from build123d import *

# Parameters (mm, degrees)
SKETCH1_R           = 8.5
SKETCH1_R_2         = 1.5
BOSS_EXTRUDE1_DEPTH = 3
FILLET1_R           = 3


with BuildPart() as part:
    # Sketch1 → Boss-Extrude1 (new body)
    with BuildSketch(Plane(origin=(0, 0, 0), x_dir=(1, 0, 0), z_dir=(0, 1, 0))):
        Polygon((-11, 0), (11, 0), (20.489621783, 17.605313925), (20.489621783, 47.605313925), (8, 62), (-8, 62), (-20.509243816, 47.910305032), (-20.509243816, 17.610706132), align=None)
        with Locations((7.519679741, 17.780252273)):
            Circle(SKETCH1_R, mode=Mode.SUBTRACT)
        with Locations((6, 4)):
            Circle(SKETCH1_R_2, mode=Mode.SUBTRACT)
        with Locations((-6, 4)):
            Circle(SKETCH1_R_2, mode=Mode.SUBTRACT)
        with Locations((-5.25, 57.999859765)):
            Circle(SKETCH1_R_2, mode=Mode.SUBTRACT)
        with Locations((5.25, 57.999859765)):
            Circle(SKETCH1_R_2, mode=Mode.SUBTRACT)
        with Locations((-13.5, 37.605313925)):
            Circle(SKETCH1_R_2, mode=Mode.SUBTRACT)
        with Locations((13.5, 37.605313925)):
            Circle(SKETCH1_R_2, mode=Mode.SUBTRACT)
        with BuildLine():
            Line((-8.730303993, 39.105313925), (8.730303993, 39.105313925))
            ThreePointArc((8.730303993, 39.105313925), (10.179901517, 41.34388933), (12.574074074, 42.518832133))
            ThreePointArc((12.574074074, 42.518832133), (0, 51.105313925), (-12.574074074, 42.518832133))
            ThreePointArc((-12.574074074, 42.518832133), (-10.179901517, 41.34388933), (-8.730303993, 39.105313925))
        make_face(mode=Mode.SUBTRACT)
        with BuildLine():
            Line((-8.730303993, 36.105313925), (8.730303993, 36.105313925))
            ThreePointArc((8.730303993, 36.105313925), (9.667400631, 34.394210987), (11.187975781, 33.171969363))
            ThreePointArc((11.187975781, 33.171969363), (11.998189223, 31.105465162), (10.062695821, 30.018841621))
            ThreePointArc((10.062695821, 30.018841621), (-0.366780245, 27.478383479), (-4.980318958, 17.785955551))
            ThreePointArc((-4.980318958, 17.785955551), (-9.241131059, 13.528058523), (-13.5, 17.787899155))
            Line((-13.5, 17.787899155), (-13.5, 32.605313925))
            ThreePointArc((-13.5, 32.605313925), (-10.541960108, 33.574185051), (-8.730303993, 36.105313925))
        make_face(mode=Mode.SUBTRACT)
    extrude(amount=BOSS_EXTRUDE1_DEPTH)

    # Fillet1
    fillet1_edges = [part.edges().sort_by_distance(p)[0] for p in [
        (-20.509243816, 1.5, -17.610706132),
        (-20.509243816, 1.5, -47.910305032),
        (-8, 1.5, -62),
        (8, 1.5, -62),
        (20.489621783, 1.5, -47.605313925),
        (20.489621783, 1.5, -17.605313925),
    ]]
    fillet(fillet1_edges, radius=FILLET1_R)


solid = part.part
The model under review builds one solid part; all positions refer to its coordinate system, in mm. A direction names the side the tool comes from. Round coordinates to 2 decimals unless told otherwise and drop trailing zeros. Order: outer loops, then holes, each group sorted by start corner. A loop starts at its lowest first (then second) coordinate and runs counter-clockwise, first axis right, second up. Notation, with made-up numbers: (-25.75, 43.5) -> (10.25, 43.5) arc R17 cw to (10.25, 62.5) -> close; hole circle Ø11 at (62, 18). An arc over 180 degrees is marked (long way). Write item = value, one per line. Start each with the question number.
Item 1: Consider section D-D on y = 1.3. Count the separate pieces of the cut face and the enclosed holes in it, plus the area to 3 significant figures.
Item 2: For faces 1 (the face through (0, 1, -62)), 2 (the face through (-0.246, 1.479, -27.576)), list the 3-axis set-ups (+Z, -Z, +X, -X, +Y, -Y) from which the entire face can be reached by the end or side of a thin tool; tool diameter is ignored.
Item 3: Consider section A-A on z = -4. Write out the cut boundary in (x, y).
Item 4: Consider section C-C on z = -12.5. Write out the cut boundary in (x, y).
Item 5: For line 1 along Z through (x, y) = (1.5, 0.5); line 2 along Z through (x, y) = (11.5, 0.55); line 3 along X through (y, z) = (1.7, -25), list the stretches that pass through material, from the lowest coordinate up.
Item 6: Consider section B-B on x = -6. Write out the cut boundary in (y, z).
Item 7: Mouldability with a two-part tool opening along X and no side actions: class faces 3 (the face through (0, 3, -38)), 4 (the face through (-10.578, 1.479, -33.548)), 5 (the face through (-20.415, 1.521, -17.624)) as released by +X, released by -X, zero draft, split by the parting line, or undercut.
Conclusion:
q1.separate_pieces = 1
q1.enclosed_holes = 9
q1.area = 1,400 mm2
q2.face_1 = -Z, +X, -X, +Y, -Y
q2.face_2 = +Y, -Y
q3.outline = (-13.16, 0) -> (-7.5, 0) -> (-7.5, 3) -> (-13.16, 3) -> close; (-4.5, 0) -> (4.5, 0) -> (4.5, 3) -> (-4.5, 3) -> close; (7.5, 0) -> (13.16, 0) -> (13.16, 3) -> (7.5, 3) -> close
q4.outline = (-17.75, 0) -> (0.86, 0) -> (0.86, 3) -> (-17.75, 3) -> close; (14.18, 0) -> (17.74, 0) -> (17.74, 3) -> (14.18, 3) -> close
q5.line_1 = -62 to -51.02, -39.11 to -36.11, -28.74 to -23.78, -11.78 to 0
q5.line_2 = -57.97 to -44.68, -42.19 to -32.96, -30.38 to -25.29, -10.27 to -0.93
q5.line_3 = -20.51 to -13.5, -2.68 to 3.03, 12.01 to 20.49
q6.outline = (0, -62) -> (3, -62) -> (3, -59.3) -> (0, -59.3) -> close; (0, -56.7) -> (3, -56.7) -> (3, -49.7) -> (0, -49.7) -> close; (0, -39.11) -> (3, -39.11) -> (3, -36.11) -> (0, -36.11) -> close; (0, -15.02) -> (3, -15.02) -> (3, -5.5) -> (0, -5.5) -> close; (0, -2.5) -> (3, -2.5) -> (3, 0) -> (0, 0) -> close
q7.face_3 = zero draft
q7.face_4 = undercut
q7.face_5 = released by -X
